Could you check a few things on this model? Use its own coordinates, in mm. A direction names the side the tool comes from. Round coordinates to 2 decimals unless told otherwise and drop trailing zeros. Write each loop counter-clockwise with the first axis right and the second up, starting at its lowest first coordinate (ties: lowest second). Pieces come first, ordered by that corner, then holes. Notation, with made-up numbers: M -12.75,58.5 L 45.25,58.5 A22 ccw 45.25,72.5 Z; hole C 37,-4.5 d10. An arc over 180 degrees is marked long. One line per item, written item: value. Start each with the question number.
(1) Thinking about a two-plate mould opening in X: for faces 4 (the face through (9, 9, -0.271)), 5 (the face through (-0.14, 17.25, 0.37)), 6 (the face through (9, 7, 4)), 7 (the face through (40, 3, 1)), which applies, released by +X, released by -X, zero draft, split by the parting line, or undercut?
(2) I want a section at B-B on z = 3.75. Please give me the cut outline in (x, y).
(3) I want a section at D-D on z = 8. Please give me the cut outline in (x, y).
(4) Which directions (+Z, -Z, +X, -X, +Y, -Y) give clear straight access to the entire face, cutting with the end or side of a thin tool? Please do faces 1 (the face through (-7, 10, 1)), 2 (the face through (-40, 15, 1)), 3 (the face through (0, 3, 9)).
(5) I'm going to push flat-ended pins straight in: pin 1 Ø4 at (x, z) = (-4.5, 10.5) entering from -Y; pin 2 Ø4 at (x, y) = (-25, 9) entering from -Z; pin 3 Ø9 at (x, y) = (22, 9.5) entering from +Z; pin 4 Ø0.6 at (y, z) = (4.5, 0.5) entering from -X. Where does each tip first touch, or does it pass through?
(6) I want a section at A-A on x = 0. Please give me the cut outline in (y, z), and give its area (3 significant figures).
(7) I want a section at C-C on x = 25. Please give me the cut outline in (y, z).
(8) If I drill on L1, parallel to Y at x = -25, z = 0.65; L2, parallel to Z at x = -27, y = 1.5; L3, parallel to X at y = 3.25, z = 0.5, over which ranges is the centre line in solid material (lowest first)?
```python
from build123d import *

# Parameters (mm, degrees)
BOSS_EXTRUDE1_DEPTH            = 15
CHAMFER1_SIZE                  = 1.802121321
CHAMFER2_SIZE                  = 1.802121321
CUT_EXTRUDE1_REACH             = 26.607
BOSS_EXTRUDE2_DEPTH            = 2.271122456
CUT_EXTRUDE2_REACH             = 52.66
F_4_2_4_2_DIAMETER_HOLE1_D     = 4.2
F_4_2_4_2_DIAMETER_HOLE1_DEPTH = 16.017925233
F_4_2_4_2_DIAMETER_HOLE2_D     = 4.2
F_4_2_4_2_DIAMETER_HOLE2_DEPTH = 16.017925233
F_5_0_5_DIAMETER_HOLE1_D       = 5
F_5_0_5_DIAMETER_HOLE2_D       = 5


with BuildPart() as part:
    # Sketch1 → Boss-Extrude1 (new body)
    with BuildSketch(Plane(origin=(0, 18, 0), x_dir=(1, 0, 0), z_dir=(0, 1, 0))):
        with BuildLine():
            Line((14, -6.5), (14, -2))
            Line((14, -2), (-14, -2))
            Line((-14, -2), (-14, -6.5))
            Line((-14, -6.5), (-5.822354851, -12.337757006))
            ThreePointArc((-5.822354851, -12.337757006), (-2.456495727, -13.897392525), (-0.156010119, -16.807587804))
            Line((-0.156010119, -16.807587804), (14, -6.5))
        make_face()
    extrude(amount=-BOSS_EXTRUDE1_DEPTH)

    # Sketch2 → Hole1 (revolve, cut)
    with BuildSketch(Plane(origin=(0, 11, 16.807587804), x_dir=(0, -1, 0), z_dir=(1, 0, 0))):
        Polygon((0, 0), (0, 10.007587804), (2, 10.007587804), (2.69979871, 0), align=None)
    revolve(axis=Axis((0, 11, -93.192412196), (0, 0, 1)), mode=Mode.SUBTRACT)

    # Chamfer1
    # the kernel refuses this chamfer: 1.802121321, 1.16968541 mm, written as the material it takes off along each edge
    with BuildSketch(Plane(origin=(-0.156010119, 12.956909278, 16.807587804), x_dir=(0.8084016240923299, 0, -0.5886313057975113), z_dir=(0, -1, 0))) as chamfer1_piece_1:
        with BuildLine():
            Line((CHAMFER1_SIZE, 0), (0.14359278, -1.207644556))
            ThreePointArc((0.14359278, -1.207644556), (0.096853733, -0.618716026), (0, 0))
            Line((0, 0), (CHAMFER1_SIZE, 0))
        make_face()
    extrude(amount=14.60910591, mode=Mode.SUBTRACT)

    # Chamfer2
    # the kernel refuses this chamfer: 1.802121321, 1.16968541 mm, written as the material it takes off along each edge
    with BuildSketch(Plane(origin=(-0.156010119, 22.652196632, 16.807587804), x_dir=(0.8084016240923299, 0, -0.5886313057975113), z_dir=(0, -1, 0))) as chamfer2_piece_1:
        with BuildLine():
            Line((CHAMFER2_SIZE, 0), (0.14359278, -1.207644556))
            ThreePointArc((0.14359278, -1.207644556), (0.096853733, -0.618716026), (0, 0))
            Line((0, 0), (CHAMFER2_SIZE, 0))
        make_face()
    extrude(amount=13.60910591, mode=Mode.SUBTRACT)

    # Chamfer3: read off the stored shape, not the designer's step
    # Chamfer3 outline → Chamfer3 (revolve, cut)
    with BuildSketch(Plane.XZ.offset(-11)):
        Polygon((2.555864922, 15.746802777), (2.555864922, 14.749238727), (3.625621395, 15.746802777), align=None)
    revolve(axis=Axis((0, 11, 0), (0, 0, 1)), mode=Mode.SUBTRACT)

    # Sketch4 → Cut-Extrude1 (cut, up to next)
    with BuildSketch(Plane.XY.offset(6.5), mode=Mode.PRIVATE) as cut_extrude1_sk1:
        with BuildLine():
            Line((9, 3), (9, 11))
            ThreePointArc((9, 11), (8.121320344, 14.878679656), (5.656854249, 18))
            Line((5.656854249, 18), (-5.656854249, 18))
            ThreePointArc((-5.656854249, 18), (-8.121320344, 14.878679656), (-9, 11))
            Line((-9, 11), (-9, 3))
            Line((-9, 3), (9, 3))
        make_face()
    cut_extrude1_tool1 = extrude(cut_extrude1_sk1.sketch, amount=-CUT_EXTRUDE1_REACH, mode=Mode.PRIVATE) & part.part
    add(cut_extrude1_tool1.solids().sort_by_distance((0, 10.176322, 6.5))[0], mode=Mode.SUBTRACT)

    # Sketch5 → Boss-Extrude2 (add)
    with BuildSketch(Plane.XY.offset(2)):
        with BuildLine():
            Line((-6.25, 0), (-6.25, 11))
            ThreePointArc((-6.25, 11), (0, 17.25), (6.25, 11))
            Line((6.25, 11), (6.25, 0))
            Line((6.25, 0), (38, 0))
            ThreePointArc((38, 0), (39.414213562, 0.585786438), (40, 2))
            Line((40, 2), (40, 4))
            ThreePointArc((40, 4), (45, 9), (40, 14))
            Line((40, 14), (40, 16))
            ThreePointArc((40, 16), (39.414213562, 17.414213562), (38, 18))
            Line((38, 18), (-38, 18))
            ThreePointArc((-38, 18), (-39.414213562, 17.414213562), (-40, 16))
            Line((-40, 16), (-40, 14))
            ThreePointArc((-40, 14), (-45, 9), (-40, 4))
            Line((-40, 4), (-40, 2))
            ThreePointArc((-40, 2), (-39.414213562, 0.585786438), (-38, 0))
            Line((-38, 0), (-6.25, 0))
        make_face()
    extrude(amount=-BOSS_EXTRUDE2_DEPTH)

    # Sketch6 → Cut-Extrude2 (cut, up to next)
    with BuildSketch(Plane(origin=(0, 0, 1), x_dir=(-1, 0, 0), z_dir=(0, 0, -1)), mode=Mode.PRIVATE) as cut_extrude2_sk1:
        with BuildLine():
            Line((-9, 11), (-9, 0))
            Line((-9, 0), (-6.25, 0))
            Line((-6.25, 0), (-6.25, 11))
            ThreePointArc((-6.25, 11), (0, 17.25), (6.25, 11))
            Line((6.25, 11), (6.25, 0))
            Line((6.25, 0), (9, 0))
            Line((9, 0), (9, 11))
            ThreePointArc((9, 11), (8.121320344, 14.878679656), (5.656854249, 18))
            Line((5.656854249, 18), (-5.656854249, 18))
            ThreePointArc((-5.656854249, 18), (-8.121320344, 14.878679656), (-9, 11))
        make_face()
    cut_extrude2_tool1 = extrude(cut_extrude2_sk1.sketch, amount=-CUT_EXTRUDE2_REACH, mode=Mode.PRIVATE) & part.part
    add(cut_extrude2_tool1.solids().sort_by_distance((7.891615, 14.768974, 1))[0], mode=Mode.SUBTRACT)

    # Ø4.2 (4.2) Diameter Hole1
    with Locations(Plane(origin=(0, 0, -0.271122456), x_dir=(-1, 0, 0), z_dir=(0, 0, -1))):
        with Locations((25, 9)):
            Hole(F_4_2_4_2_DIAMETER_HOLE1_D / 2, depth=F_4_2_4_2_DIAMETER_HOLE1_DEPTH)

    # Ø4.2 (4.2) Diameter Hole2
    with Locations(Plane(origin=(0, 0, -0.271122456), x_dir=(-1, 0, 0), z_dir=(0, 0, -1))):
        with Locations((-25, 9)):
            Hole(F_4_2_4_2_DIAMETER_HOLE2_D / 2, depth=F_4_2_4_2_DIAMETER_HOLE2_DEPTH)

    # Ø5.0 (5) Diameter Hole1 (through all)
    with Locations(Plane.XY.offset(2)):
        with Locations((40, 9)):
            Hole(F_5_0_5_DIAMETER_HOLE1_D / 2)

    # Ø5.0 (5) Diameter Hole2 (through all)
    with Locations(Plane.XY.offset(2)):
        with Locations((-40, 9)):
            Hole(F_5_0_5_DIAMETER_HOLE2_D / 2)


solid = part.part
```
Found:
1. face 4: zero draft
1. face 5: undercut
1. face 6: undercut
1. face 7: released by +X
2. outline: M -14,3 L -9,3 L -9,11 A9 cw -5.66,18 L -14,18 Z; M 5.66,18 A9 cw 9,11 L 9,3 L 14,3 L 14,18 Z
3. outline: M -11.9,3 L 11.94,3 L 11.94,18 L -11.9,18 Z; hole C 0,11 d4.17
4. face 1: -Y
4. face 2: +Z, -Z, -X, +Y
4. face 3: +Z, +X, -X, -Y
5. pin 1: stops at y = 3
5. pin 2: passes through
5. pin 3: stops at z = 2
5. pin 4: stops at x = -42.71
6. outline: M 3,6.5 L 18,6.5 L 18,15.75 L 14.63,15.75 L 13.56,14.75 L 13,6.8 L 9,6.8 L 8.44,14.75 L 7.37,15.75 L 3,15.75 Z; M 17.25,-0.27 L 18,-0.27 L 18,1 L 17.25,1 Z
6. area: 97.3 mm²
7. outline: M 0,-0.27 L 6.9,-0.27 L 6.9,2 L 0,2 Z; M 11.1,-0.27 L 18,-0.27 L 18,2 L 11.1,2 Z
8. L1: y = 0 to 6.9, 11.1 to 18
8. L2: z = -0.27 to 2
8. L3: x = -40 to -6.25, 6.25 to 40
